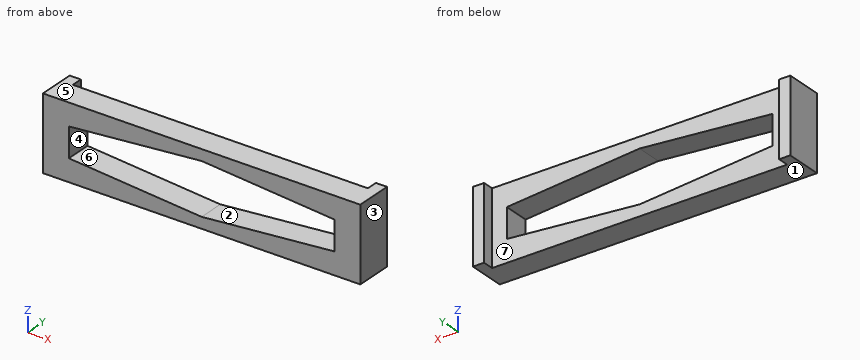
Autodesk Inventor part; units mm, degrees
ref_plane "YZ Plane" through (0, 0, 0) normal (1, 0, 0) x (0, 1, 0)
ref_plane "XZ Plane" through (0, 0, 0) normal (0, 1, 0) x (-1, 0, 0)
ref_plane "XY Plane" through (0, 0, 0) normal (0, 0, 1) x (1, 0, 0)
sketch "Sketch1" plane through (0, 0, 0) normal (0, 1, 0) x (-1, 0, 0)
  line L0 (0, 0) -> (0, 38)
  line L1 (0, 38) -> (0, 43)
  line L2 (0, 38) -> (2, 38)
  line L3 (2, 38) -> (-2, 38)
  line L4 (-2, 38) -> (0, 43)
  line L5 (2, 38) -> (0, 43)
  line L6 (-2, 38) -> (-2, 2)
  line L7 (2, 2) -> (2, 38)
  line L8 (-2, 2) -> (-2, 3)
  line L9 (2, 2) -> (2, 0)
  line L10 (-2, 2) -> (-2, 0)
  line L11 (-2, 0) -> (2, 0)
  line L12 (0, 0) -> (-2, 1)
  line L13 (0, 38) -> (0, 42)
  line L14 (0, 42) -> (-0.4, 42)
  line L15 (0.4, 42) -> (0, 42)
  line L16 (0, 0) -> (0, 10)
  line L17 (0, 10) -> (0, 0)
  line L18 (0, 0) -> (-40, 0)
  line L19 (-40, 0) -> (-40, -10)
  line L20 (-40, 10) -> (40, 10)
  line L21 (40, 10) -> (40, -10)
  line L22 (40, -10) -> (-40, -10)
  line L23 (-40, -10) -> (-40, 10)
  line L24 (40, -10) -> (38, -10)
  line L25 (38, -10) -> (43, -10)
  line L26 (43, -10) -> (43, 10)
  line L27 (43, 10) -> (38, 10)
  line L28 (38, 10) -> (38, -10)
  line L29 (-40, -10) -> (-38, -10)
  line L30 (-38, -10) -> (-43, -10)
  line L31 (-43, -10) -> (-43, 10)
  line L32 (-43, 10) -> (-38, 10)
  line L33 (-38, 10) -> (-38, -10)
  point P0 (0, 2)
  dimension "d0" = 38
  dimension "d1" = 5
  dimension "d2" = 2
  dimension "d3" = 4
  dimension "d6" = 1
  dimension "d30" = 4
  dimension "d31" = 10
  dimension "d32" = 40
  dimension "d33" = 10
  dimension "d34" = 80
  dimension "d37" = 2
  dimension "d38" = 5
  dimension "d39" = 2
  dimension "d40" = 5
extrude "Extrusion1" add sketch "Sketch1" along normal blind 7 contours L12 L10 L6 L20 L0 | L11 L9 L7 L20 L28 L22 L33 L18 | L0 L20 L7 L9 L11 | L11 L10 L12 | L18 L33 L20 L6 L10 | L33 L22 L19 L18 | L18 L23 L20 L33 | L20 L21 L22 L28 | L19 L30 L31 L32 L23 | L27 L26 L25 L21
sketch "Sketch4" plane through (0, 7, 0) normal (0, 1, 0) x (1, 0, 0)
  circle A0 centre (0, 0) radius 1.5
  line L0 (0, 0) -> (-36, 0)
  line L1 (-36, 0) -> (-36, -4)
  line L2 (0, 0) -> (0, -7)
  line L3 (-36, -4) -> (0, -7)
  line L4 (-36, 0) -> (-36, 4)
  line L5 (0, 0) -> (0, 7)
  line L6 (-36, 4) -> (0, 7)
  line L7 (0, 0) -> (36, 0)
  line L8 (36, 0) -> (36, -4)
  line L9 (36, -4) -> (0, -7)
  line L10 (36, 4) -> (0, 7)
  line L11 (36, 0) -> (36, 4)
  dimension "d20" = 3
  dimension "d26" = 36
  dimension "d28" = 4
  dimension "d29" = 7
extrude "Extrusion5" cut sketch "Sketch4" against normal through all
extrude "Extrusion6" add sketch "Sketch1" along normal blind 3 from surface at 7 contours L19 L30 L31 L32 L23 | L27 L26 L25 L21
properties part number "testing deadbolt arm adapter"
Geometry check sheet. Reference: the model listing, model coordinates, mm. Face numbers are marked on the shaded views. A direction names the side the tool comes from. Give positions to 0.01 mm unless a question says otherwise; leave off trailing zeros. Loops run counter-clockwise (first coordinate to the right, second up) from the corner with the lowest first, then second, coordinate; pieces in that order, holes last. Notation, with made-up numbers: M 66.25,77 L 122.25,77 A23 cw 122.25,91 Z; hole C -23,17.25 d1. An arc over 180 degrees is marked long. Answer as a JSON object with one key per item and string values. Group by question number.
Item 1: Sectioned sample at A-A on z = 0.5. Record the boundary of the cut face in (x, y).
Item 2: Sectioned sample at C-C on x = -10. Record the boundary of the cut face in (y, z).
Item 3: Sectioned sample at D-D on z = 6. Record the boundary of the cut face in (x, y), plus the area to 3 significant figures.
Item 4: Access from +Z, -Z, +X, -X, +Y, -Y to the whole of each face (thin tool, end or side, straight path). Record for the marked faces 5, 6 and 7.
Item 5: Mould release check, pull along X, two halves, no side actions. Record for the marked faces 1, 2, 3 and 4: pulls with the +X half, pulls with the -X half, needs draft (parallel to the pull), parting line crosses it, or undercut.
Item 6: Sectioned sample at B-B on y = 5. Record the boundary of the cut face in (x, z), plus the area to 3 significant figures.
Item 7: Gauge pin test, flat end, axial feed: pin 1 (6 mm diameter, centred on x = -14, z = 3, fed in from +Y). Record the tip position at first contact, or that the pin passes through.
Item 8: Material ranges on L1, parallel to X at y = 4, z = -3.75; L2, parallel to X at y = 9, z = 7.75; L3, parallel to Y at x = -4.5, z = -7.75, recorded low to high.
Findings below:
{
 "1": {"outline": "M -43,0 L -36,0 L -36,7 L -40,7 L -40,10 L -43,10 Z; M 36,0 L 43,0 L 43,10 L 40,10 L 40,7 L 36,7 Z"},
 "2": {"outline": "M 0,-10 L 7,-10 L 7,-6.17 L 0,-6.17 Z; M 0,6.17 L 7,6.17 L 7,10 L 0,10 Z"},
 "3": {"outline": "M -43,0 L -12,0 L -12,7 L -40,7 L -40,10 L -43,10 Z; M 12,0 L 43,0 L 43,10 L 40,10 L 40,7 L 12,7 Z", "area": "452 mm2"},
 "4": {"face 5": "+Z, +X, -X, +Y, -Y", "face 6": "+Y, -Y", "face 7": "+Z, -Z, +Y"},
 "5": {"face 1": "needs draft", "face 2": "undercut", "face 3": "pulls with the +X half", "face 4": "undercut"},
 "6": {"outline": "M -43,-10 L 43,-10 L 43,10 L -43,10 Z; hole M -36,-4 L 0,-7 L 36,-4 L 36,4 L 0,7 L -36,4 Z", "area": "928 mm2"},
 "7": {"pin 1": "y = 7"},
 "8": {"L1": "-43 to -36, 36 to 43", "L2": "-43 to -40, 40 to 43", "L3": "0 to 7"}
}
